```python
from build123d import *

# Parameters (mm, degrees)
CROQUIS3_R            = 4.7625
CORTAR_EXTRUIR2_DEPTH = 10


with BuildPart() as part:
    # Croquis2 → Revolución1 (revolve)
    with BuildSketch(Plane.XY):
        with BuildLine():
            Line((40, 0), (60, 0))
            Line((60, 0), (60, 5))
            Line((60, 5), (43.547405025, 5))
            Line((43.547405025, 5), (28.266159728, 48.660700849))
            ThreePointArc((28.266159728, 48.660700849), (27.535723945, 49.631165488), (26.378443015, 50))
            Line((26.378443015, 50), (25.31896201, 50))
            ThreePointArc((25.31896201, 50), (23.687796522, 49.15728093), (23.431245297, 47.339299151))
            Line((23.431245297, 47.339299151), (40, 0))
        make_face()
    revolve(axis=Axis((0, 0, 0), (0, 1, 0)))

    # Croquis3 → Cortar-Extruir2 (cut)
    with BuildSketch(Plane.XZ):
        with Locations((0, 50)):
            Circle(CROQUIS3_R)
        with Locations((43.301270189, -25)):
            Circle(CROQUIS3_R)
        with Locations((-43.301270189, -25)):
            Circle(CROQUIS3_R)
    extrude(amount=-CORTAR_EXTRUIR2_DEPTH, mode=Mode.SUBTRACT)


solid = part.part
```
The listing builds one solid part. Answer for the finished solid, in the listing's coordinates (mm). A direction names the side the tool comes from. Give positions to 0.01 mm unless a question says otherwise; leave off trailing zeros. Order: outer loops, then holes, each group sorted by start corner. A loop starts at its lowest first (then second) coordinate and runs counter-clockwise, first axis right, second up. Notation, with made-up numbers: M 68.5,43 L 93.5,43 A24 ccw 93.5,67 Z; hole C -38,60 d1. An arc over 180 degrees is marked long. Put each result on its own line as item: value. Start each with the question number.
Item 1: Which of the six approach directions +Z, -Z, +X, -X, +Y, -Y give full straight-line access (tool end or side, diameter ignored) to faces 1 (the face through (-6.1, 33.86, 27.48)), 2 (the face through (-18, 5, 40))?
Item 2: The part is cut by section C-C, the plane y = 42. Determine the outline of the cut face in (x, z), and give its area (3 significant figures).
Item 3: Flat-ended cylindrical pins translate along their axes: P1, Ø11, axis at x = 43.3, z = -25, coming from the +Y side; P2, Ø8, axis at x = -26, y = 15.5, coming from the +Z side; P3, Ø3, axis at x = 18.5, y = 27, coming from the +Z side. Find the tip coordinate at first contact, or state that the pin passes through.
Item 4: The part is cut by section B-B, the plane z = 50. Determine the outline of the cut face in (x, y), and give its area (3 significant figures).
Item 5: For a pull along Z with two mould halves and no side action, classify faces 3 (the face through (-25.71, 36.84, 19.72)), 4 (the face through (-3.51, 2.46, 53.22)), 5 (the face through (-39, 0, 12)) as +Z half, -Z half, draft (parallel to the pull), parting line (faces both ways), or undercut.
Item 6: The part is cut by section D-D, the plane z = 0. Determine the outline of the cut face in (x, y), and give its area (3 significant figures).
Item 7: The part is cut by section A-A, the plane x = 0. Determine the outline of the cut face in (y, z), and give its area (3 significant figures).
Item 8: Find the intervals of material crossed by line 1 along Z through (x, y) = (0, 1); line 2 along Y through (x, z) = (-25, 53); line 3 along X through (y, z) = (27.5, 22), in increasing order.
Answer key:
1. face 1: -Y
1. face 2: +Y
2. outline: C 0,0 d61.19; hole C 0,0 d50.6
2. area: 930 mm²
3. P1: stops at y = 5
3. P2: stops at z = 33.74
3. P3: stops at z = 31.76
4. outline: M -33.17,0 L -4.76,0 L -4.76,5 L -33.17,5 Z; M 4.76,0 L 33.17,0 L 33.17,5 L 4.76,5 Z
4. area: 284 mm²
5. face 3: parting line
5. face 4: undercut
5. face 5: draft
6. outline: M -60,0 L -40,0 L -23.43,47.34 A2 ccw -25.32,50 L -26.38,50 A2 ccw -28.27,48.66 L -43.55,5 L -60,5 Z; M 23.43,47.34 L 40,0 L 60,0 L 60,5 L 43.55,5 L 28.27,48.66 A2 ccw 26.38,50 L 25.32,50 A2 ccw Z
6. area: 681 mm²
7. outline: M 0,-60 L 5,-60 L 5,-43.55 L 48.66,-28.27 A2 ccw 50,-26.38 L 50,-25.32 A2 ccw 47.34,-23.43 L 0,-40 Z; M 0,40 L 47.34,23.43 A2 ccw 50,25.32 L 50,26.38 A2 ccw 48.66,28.27 L 5,43.55 L 5,45.24 L 0,45.24 Z; M 0,54.76 L 5,54.76 L 5,60 L 0,60 Z
7. area: 634 mm²
8. line 1: z = -60 to -39.65, 39.65 to 45.24, 54.76 to 60
8. line 2: y = 0 to 5
8. line 3: x = -28.08 to -20.94, 20.94 to 28.08
